from build123d import *

# Parameters (mm, degrees)
F2_W     = 90
F2_H     = 99
F3_DEPTH = 60


with BuildPart() as f1:
    # F0 (on Front) → F1 (revolve)
    with BuildSketch(Plane.XZ):
        with BuildLine():
            Line((28.5875385463, 3.7629891087), (28.5875385463, -36.5419039394))
            add(Edge.make_bspline(
                [(28.5875385463, -36.5419039394), (36.877758444, -36.5419039394), (38.6275867194, -35.8378488567), (39.3034274749, -27.6489692273), (52.7312499665, -28.0489931449), (55.7562974133, -9.2624192261), (57.687700038, 3.7629891087)],
                knots=[0, 0, 0, 0, 0.2273966772, 0.3897712394, 0.6048240119, 1, 1, 1, 1], degree=3))
            Line((57.687700038, 3.7629891087), (28.5875385463, 3.7629891087))
        make_face()
    revolve(axis=Axis((28.5875385463, 0, -16.3894574153), (0, 0, 1)))


with BuildPart() as f3:
    # F2 (on Front) → F3 (new body)
    with BuildSketch(Plane.XZ):
        with Locations((26.7319735885, -9.2539225817)):
            Rectangle(F2_W, F2_H)
    extrude(amount=-F3_DEPTH)

    # F4: cut F1
    add(f1.part, mode=Mode.SUBTRACT)


solid = f3.part
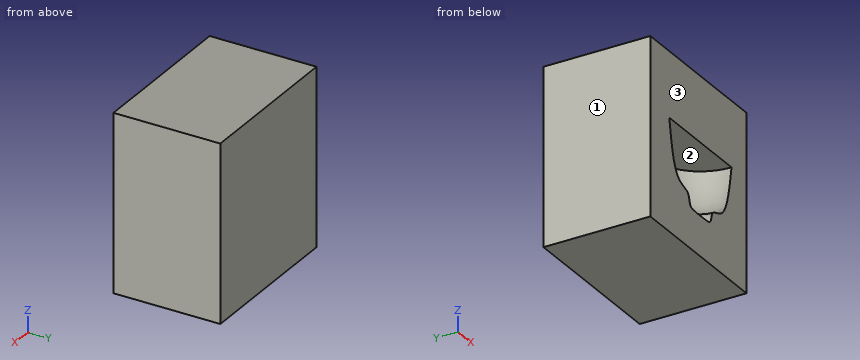
Geometry: final body of the model. Coordinates: model frame, mm. Face numbers are marked on the shaded views. Coordinates: 2 decimals unless noted, no trailing zeros. Use one line per item in the form item = value.
1) Mould query, pull axis X, two halves, no side actions, for the marked faces 1, 2 and 3. Classes: +X half, -X half, draft (parallel to the pull), parting line (faces both ways), or undercut.
Solutions:
face_1 = -X half
face_2 = undercut
face_3 = draft
2) Pin query (flat end, axial travel): pin 1 (2 mm diameter, centred on x = 11, z = 2, fed in from -Y). Return the tip coordinate at first contact, or that it passes through.
Solutions:
pin_1 = 22.03
3) Ray query, L1, parallel to Z at x = 52, y = 6; L2, parallel to X at y = 10.5, z = -3; L3, parallel to X at y = 15.5, z = -20.5. Return the intervals inside material, ascending.
Solutions:
L1 = -58.75 to -19.27, 3.76 to 40.25
L2 = -18.27 to 2.57, 54.61 to 71.73
L3 = -18.27 to 10.73, 46.45 to 71.73
